from build123d import *

# Parameters (mm, degrees)
FILLET1_R   = 0.6
HEX_2_DEPTH = 3.0988


with BuildPart() as part:
    # BodySke → BaseBody (revolve)
    with BuildSketch(Plane.XY):
        with BuildLine():
            Line((68.8, 0), (68.8, 6.8985))
            Line((68.8, 6.8985), (67.6985, 8))
            Line((67.6985, 8), (8.8, 8))
            Line((8.8, 8), (8.8, 14))
            Line((8.8, 14), (8.42, 14))
            ThreePointArc((8.42, 14), (3.53447189, 11.312563812), (0, 7))
            Line((0, 7), (0, 0))
            Line((0, 0), (68.8, 0))
        make_face()
    revolve(axis=Axis((0, 0, 0), (1, 0, 0)))

    # Fillet1
    fillet1_edges = [part.edges().sort_by_distance(p)[0] for p in [
        (8.8, -8, 0),
    ]]
    fillet(fillet1_edges, radius=FILLET1_R)

    # Sketch2 → PreBroach (revolve, cut)
    with BuildSketch(Plane.XY):
        Polygon((0, 5), (3.0988, 5), (5.985551346, 0), (0, 0), align=None)
    revolve(axis=Axis((0, 0, 0), (1, 0, 0)), mode=Mode.SUBTRACT)

    # Sketch3 → Hex 2 (cut)
    with BuildSketch(Plane(origin=(0, 0, 0), x_dir=(0, 0, -1), z_dir=(1, 0, 0))):
        Polygon((-5, -2.886751346), (-5, 2.886751346), (0, 5.773502692), (5, 2.886751346), (5, -2.886751346), (0, -5.773502692), align=None)
    extrude(amount=HEX_2_DEPTH, mode=Mode.SUBTRACT)


solid = part.part
Input: part model. Units: mm. Frame: model coordinates. A direction names the side the tool comes from. Give positions to 0.01 mm unless a question says otherwise; leave off trailing zeros. Loops run counter-clockwise (first coordinate to the right, second up) from the corner with the lowest first, then second, coordinate; pieces in that order, holes last. Notation, with made-up numbers: M 19,30 L 41,30 A21 cw 41,44 Z; hole C 27.25,68 d11. An arc over 180 degrees is marked long. Use one line per item in the form item = value.
1. Line query: L1, parallel to Z at x = 33, y = -0.5; L2, parallel to X at y = 10.25, z = 1.5; L3, parallel to Y at x = 22, z = -1.75. Output: solid intervals per line, ascending.
Numbers:
L1 = -7.98 to 7.98
L2 = 2.49 to 8.8
L3 = -7.81 to 7.81
2. Reachability of faces 5 (the face through (3.099, 5.2, 0)), 6 (the face through (8.8, 6.4, -6)), 7 (the face through (8.607, 12.932, -5.362)) from +Z, -Z, +X, -X, +Y, -Y: full face, straight path, thin tool, end or side. Return the list, or none.
Numbers:
face_5 = -X
face_6 = +X
face_7 = +X, -X
3. Section query B-B, the plane y = -10. Return the cut outline in (x, z).
Numbers:
outline = M 8.42,-9.8 L 8.8,-9.8 L 8.8,9.8 L 8.42,9.8 A10.79 ccw Z
4. Pull-direction query (Z, two-part tool) for faces 1 (the face through (0, -5, -2)), 2 (the face through (3.099, 2.7, -4.5)), 3 (the face through (1.528, -4.31, -2.535)), 4 (the face through (38.14, -1.73, -7.81)); classes: released by +Z, released by -Z, zero draft, split by the parting line, or undercut.
Numbers:
face_1 = zero draft
face_2 = undercut
face_3 = undercut
face_4 = split by the parting line
5. Section query A-A, the plane x = 23. Return the cut outline in (y, z).
Numbers:
outline = C 0,0 d16
6. First-contact query: pin 1 (8 mm diameter, centred on x = 20.5, y = 0, fed in from +Z); pin 2 (2.5 mm diameter, centred on y = 2, z = 3.5, fed in from -X); pin 3 (2.5 mm diameter, centred on x = 1.5, y = 1.5, fed in from -Z); pin 4 (3 mm diameter, centred on x = 11.5, y = -10, fed in from +Z). Flat tips, straight axial feed; report the tip coordinate or a pass-through.
Numbers:
pin_1 = 8
pin_2 = 3.1
pin_3 = -10.52
pin_4 = through
